Could you check a few things on this model? Use its own coordinates, in mm. Give positions to 0.01 mm unless a question says otherwise; leave off trailing zeros. Loops run counter-clockwise (first coordinate to the right, second up) from the corner with the lowest first, then second, coordinate; pieces in that order, holes last. Notation, with made-up numbers: (66.25, 73) -> (106.25, 73) arc R14 ccw to (106.25, 86) -> close; hole circle Ø3 at (-1.5, 29.25). An arc over 180 degrees is marked (long way). Write item = value, one per line. Start each with the question number.
1) I want a section at B-B (y = -69). List the corners of the cut face in (x, z) for me.
2) I'm going to push flat-ended pins straight in: pin 1 Ø8 at (x, z) = (-76, 32.5) entering from +Y; pin 2 Ø1.5 at (y, z) = (-25.5, 66) entering from -X; pin 3 Ø1.5 at (y, z) = (-51.5, 89.5) entering from -X. Where does each tip first touch, or does it pass through?
3) I want a section at D-D (y = 38.5). List the corners of the cut face in (x, z) for me.
4) I want a section at A-A (z = 88). List the corners of the cut face in (x, y) for me, and give its area (3 significant figures).
5) I want a section at C-C (x = -76.5). List the corners of the cut face in (y, z) for me, and give its area (3 significant figures).
6) I need wall thicknesses on probe 1 along Y at (x, z) = (-45.5, 209); probe 2 along Y at (x, z) = (82, 85); probe 3 along X at (y, z) = (25, 76). Which ranges of each line are inside material? Lowest first, please. Write a range as from..to.
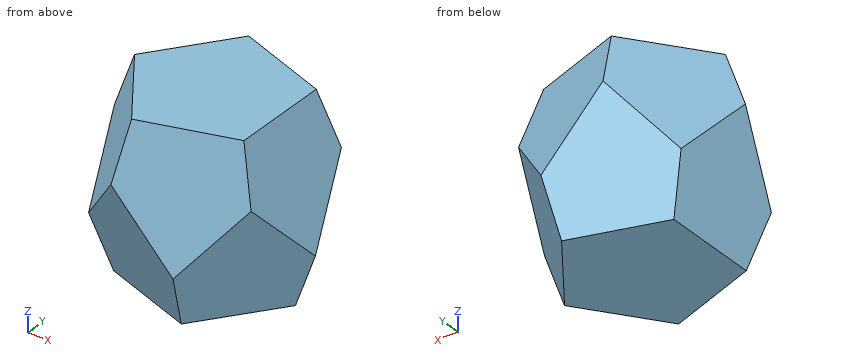
Solid Edge part; units mm, degrees
sketch "Sketch1" plane through (0, 0, 0) normal (0, -1, 0) x (1, 0, 0)
  arc A0 (0, 363.8406) -> (0, -136.1594) centre (0, 113.8406) ccw
  line L0 (0, 363.8406) -> (0, -136.1594)
revolve "RevolvedProtrusion1" add sketch "Sketch1" angle 360 about axis through (0, 0, 363.8406) along (0, 0, -1)
sketch "Sketch2" plane through (0, 0, 0) normal (0, -1, 0) x (1, 0, 0)
  line L0 (-85.0651, 0) -> (-128.677, 147.5749)
  line L1 (-85.0651, 0) -> (68.8191, 0)
extrude "Cutout1" cut sketch "Sketch2" against normal up to next and the other way up to next material side at (-106.919, 0, 73.7733)
sketch "Sketch3" plane through (0, 0, 0) normal (0, -1, 0) x (1, 0, 0)
  line L0 (-68.8191, 227.6813) -> (85.0651, 227.6813)
  line L1 (85.0651, 227.6813) -> (128.677, 80.1064)
extrude "Cutout2" cut sketch "Sketch3" against normal up to next and the other way up to next material side at (8.123, 0, 227.7313)
pattern_circular "Pattern1" count 5 over 360 about axis through (0, 0, 0) along (0, 0, 1) of "Cutout1", "Cutout2"
Answer list:
q1.outline = (-108.82, 80.38) -> (-94.97, 33.52) -> (-62.92, 0) -> (55.01, 0) -> (108.82, 147.3) -> (94.97, 194.16) -> (62.92, 227.68) -> (-55.01, 227.68) -> close
q2.pin_1 = 76.65
q2.pin_2 = -104.79
q2.pin_3 = -111.74
q3.outline = (-118.73, 113.92) -> (-85.07, 0) -> (77.17, 0) -> (118.73, 113.76) -> (85.07, 227.68) -> (-77.17, 227.68) -> close
q4.outline = (-111.07, -62.07) -> (-93.36, -86.45) -> (24.71, -124.82) -> (53.37, -115.5) -> (126.34, -15.07) -> (126.34, 15.07) -> (53.37, 115.5) -> (24.71, 124.82) -> (-93.36, 86.45) -> (-111.07, 62.07) -> close
q4.area = 44,000 mm^2
q5.outline = (-98.7, 109.79) -> (-64.59, 0) -> (64.59, 0) -> (98.7, 109.79) -> (39.43, 227.68) -> (-39.43, 227.68) -> close
q5.area = 34,200 mm^2
q6.probe_1 = -91.49..91.49
q6.probe_2 = -74.59..74.59
q6.probe_3 = -107.52..114.74
